```python
from build123d import *

# Parameters (mm, degrees)
F0_R     = 12.7
F0_R_2   = 9.525
F1_DEPTH = 406.4
F2_R     = 3.175
F3_DEPTH = 12.7
F4_R     = 3.175
F5_DEPTH = 12.7


with BuildPart() as f1:
    # F0 (on Front) → F1 (new body)
    with BuildSketch(Plane.XZ):
        Circle(F0_R)
        Circle(F0_R_2, mode=Mode.SUBTRACT)
    extrude(amount=F1_DEPTH)

    # F2 (on Right) → F3 (cut, symmetric)
    with BuildSketch(Plane.YZ):
        with Locations((-101.6, 0)):
            Circle(F2_R)
        with Locations((-76.2, 0)):
            Circle(F2_R)
    extrude(amount=F3_DEPTH, both=True, mode=Mode.SUBTRACT)

    # F4 (on Top) → F5 (cut, symmetric)
    with BuildSketch(Plane.XY):
        with Locations((0, -76.2)):
            Circle(F4_R)
        with Locations((0, -101.6)):
            Circle(F4_R)
    extrude(amount=F5_DEPTH, both=True, mode=Mode.SUBTRACT)


solid = f1.part
```
Geometry check sheet. Reference: the model listing, model coordinates, mm. Round coordinates to 2 decimals unless told otherwise and drop trailing zeros. Loops run counter-clockwise (first coordinate to the right, second up) from the corner with the lowest first, then second, coordinate; pieces in that order, holes last. Notation, with made-up numbers: (80, -27) - (122, -27) arc R18 cw to (122, -7) - close; hole circle Ø1 at (-20.5, 55.5). An arc over 180 degrees is marked (long way). Write each question's results on one line, items separated by ' | '. Start each with the question number.
Q1. Release check for a two-part mould opening along X. For faces 1 (the cylindrical face through (1.5, -104.4, 10.9)), 2 (the cylindrical face through (-2.75, -200.36, -12.4)), 3 (the cylindrical face through (-7.559, -200.355, -5.796)), 4 (the cylindrical face through (-10.81, -73.17, 0.95)) record: +X half, -X half, draft (parallel to the pull), parting line (faces both ways), or undercut.
Q2. Gauge pin test, flat ends, axial feed: P1, Ø1.5, axis at x = -8.5, y = -303.5, coming from the +Z side; P2, Ø8, axis at x = 4.5, y = -291.5, coming from the -Z side; P3, Ø10, axis at y = -76.2, z = 0, coming from the -X side; P4, Ø1.5, axis at y = -69, z = -5, coming from the +X side. Record the tip position at first contact, or that the pin passes through.
Q3. Thickness scan on line 1 (Y direction, x = 0, z = -10.95) (3 decimals); line 2 (Z direction, x = 0, y = -301) (3 decimals); line 3 (X direction, y = -387.5, z = -0.25). Record the ranges inside material, lowest first. Write a range as [from, to].
Q4. Cross-section at A-A on y = -92. Enter the section's corners in (x, z) (3 decimals), and give its area (3 significant figures).
Answers below:
1) face 1: undercut | face 2: parting line | face 3: undercut | face 4: draft
2) P1: stops at z = 10.06 | P2: stops at z = -12.69 | P3: stops at x = -12.7 | P4: stops at x = 11.97
3) line 1: y = [-406.4, -104.775], [-98.425, -79.375], [-73.025, 0] | line 2: z = [-12.7, -9.525], [9.525, 12.7] | line 3: x = [-12.7, -9.52], [9.52, 12.7]
4) outline: circle Ø25.4 at (0, 0); hole circle Ø19.05 at (0, 0) | area: 222 mm²
